Autodesk Inventor part; units mm, degrees
sketch "Esboço1" plane through (0, 0, 0) normal (0, 0, 1) x (1, 0, 0)
  arc A0 (3.678, 19.15) -> (4.657, -18.9358) centre (0, 0) ccw
  line L0 (3.678, 19.15) -> (39.7998, 12.2124)
  line L1 (57.7995, -7.9297) -> (59.2705, -26.8636)
  arc A1 (56.1556, -38.4578) -> (59.2705, -26.8636) centre (41.3246, -28.2578) ccw
  arc A2 (24.8291, -31.7542) -> (47.6703, -45.4578) centre (42.4793, -28.2226) ccw
  arc A3 (57.7995, -7.9297) -> (39.7998, 12.2124) centre (35.6, -9.6544) ccw
  line L2 (56.1556, -38.4578) -> (47.6703, -45.4578)
  arc A4 (24.8291, -31.7542) -> (4.657, -18.9358) centre (8.6077, -35) ccw
  point P0 (17.4802, -21.0376)
  point P1 (51.913, -41.9578)
  point P2 (33.2189, -43.6578)
  point P3 (58.7081, -32.928)
  point P4 (58.535, -17.3966)
  dimension "d6" = 19.5
  dimension "d30" = 8.6077
  dimension "d34" = 35
  dimension "d35" = 51
  dimension "d36" = 13.7
  dimension "d37" = 17.2
  dimension "d38" = 15.4
  dimension "d39" = 18
  dimension "d40" = 11
  dimension "d41" = 18
  dimension "d42" = 22.935
  dimension "d43" = 35.6
  dimension "d44" = 19.15
extrude "Extrusão1" add sketch "Esboço1" along normal mid plane 2
For this review, take the finished solid that the model builds, in its own axes (mm). Coordinates: 2 decimals unless noted, no trailing zeros. Order: outer loops, then holes, each group sorted by start corner. A loop starts at its lowest first (then second) coordinate and runs counter-clockwise, first axis right, second up. Notation, with made-up numbers: (60.25, 41.5) - (93.25, 41.5) arc R28 cw to (93.25, 65.5) - close; hole circle Ø8 at (4, 62.25). An arc over 180 degrees is marked (long way). Answer as a JSON object with one key per item and string values. Group by question number.
1. Clearance check with a flat-ended pin moving along its axis: P1, Ø1, axis at y = 2.5, z = 0.5, coming from the -X side. State where the tip first meets the part, or that it passes through.
2. For probe 1 along Y at (x, z) = (4, -0.4); probe 2 along X at (y, z) = (-29, -0.9); probe 3 along Y at (x, z) = (48, 0.2), list the stretches that pass through material, from the lowest coordinate up.
3. We need section A-A on z = 0.3. State the section outline as (x, y) points, then the cut area to 3 significant figures.
4. We need section B-B on x = 33. State the section outline as (y, z) points, then the cut area to 3 significant figures.
5. We need section C-C on y = 9. State the section outline as (x, z) points, then the cut area to 3 significant figures.
6. The part is to be moulded in two halves that separate along X. For faces 1 (the cylindrical face through (33.399, -43.765, -0.014)), 2 (the cylindrical face through (58.73, -32.85, -0.01)), 3 (the cylindrical face through (17.322, -20.938, -0.014)), say which applies: pulls with the +X half, pulls with the -X half, needs draft (parallel to the pull), parting line crosses it, or undercut.
Final values:
{
 "1": {"P1": "x = -19.4"},
 "2": {"probe 1": "-19.09 to 19.09", "probe 2": "24.02 to 59.31", "probe 3": "-45.19 to 8.84"},
 "3": {"outline": "(3.68, 19.15) arc R19.5 ccw (long way) to (4.66, -18.94) arc R16.54 cw to (24.83, -31.75) arc R18 ccw to (47.67, -45.46) - (56.16, -38.46) arc R18 ccw to (59.27, -26.86) - (57.8, -7.93) arc R22.27 ccw to (39.8, 12.21) - close", "area": "3,310 mm²"},
 "4": {"outline": "(-43.52, -1) - (13.52, -1) - (13.52, 1) - (-43.52, 1) - close", "area": "114 mm²"},
 "5": {"outline": "(-17.3, -1) - (47.76, -1) - (47.76, 1) - (-17.3, 1) - close", "area": "130 mm²"},
 "6": {"face 1": "parting line crosses it", "face 2": "pulls with the +X half", "face 3": "undercut"}
}
